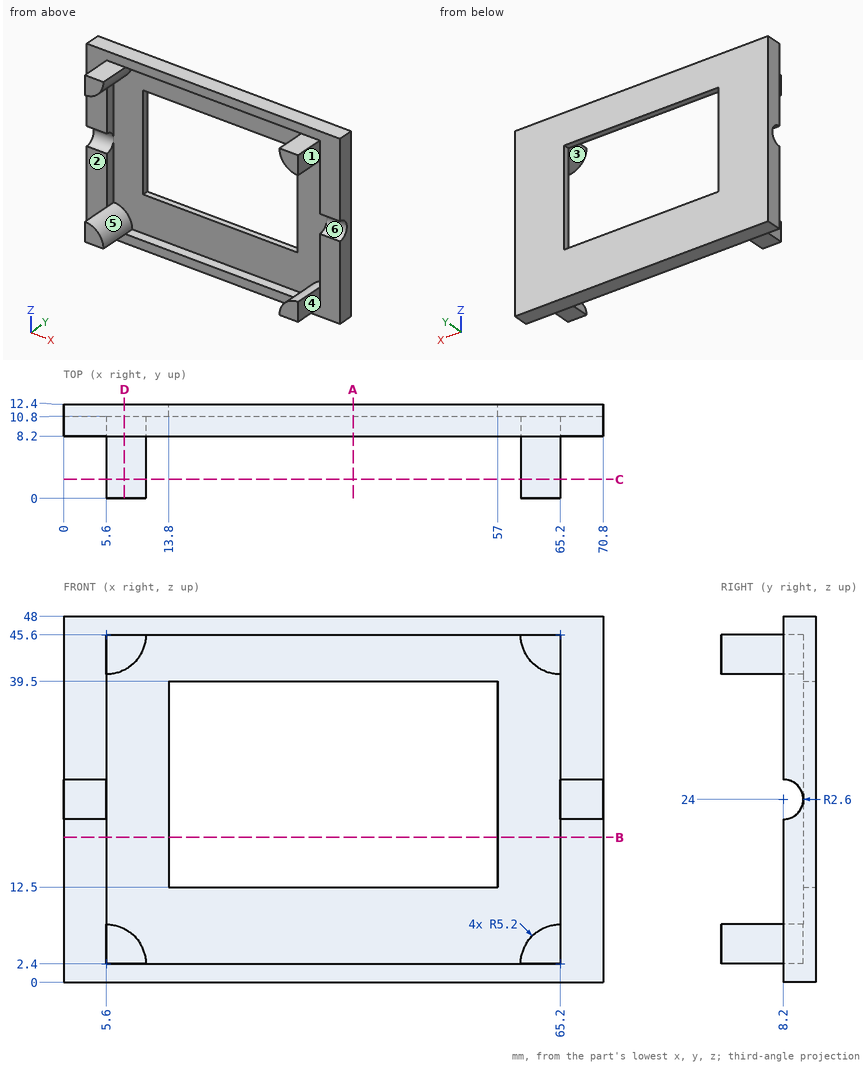
Geometry check sheet. Reference: drawing and pictorial views, mm from the part's lowest x, y, z. A direction names the side the tool comes from. Coordinates: 2 decimals unless noted, no trailing zeros. Loops run counter-clockwise (first coordinate to the right, second up) from the corner with the lowest first, then second, coordinate; pieces in that order, holes last.
1) Material ranges on probe 1 along X at (y, z) = (9.25, 29.5); probe 2 along Z at (x, y) = (44, 9.75); probe 3 along Y at (x, z) = (28, 8), recorded low to high.
2) Sectioned sample at C-C (y = 2.5). Record the boundary of the cut face in (x, z), and give its area (3 significant figures).
3) Sectioned sample at A-A (x = 38). Record the boundary of the cut face in (y, z).
4) Sectioned sample at D-D (x = 8). Record the boundary of the cut face in (y, z), and give its area (3 significant figures).
5) Access from +Z, -Z, +X, -X, +Y, -Y to the whole of each face (thin tool, end or side, straight path). Record for the marked faces 4, 5 and 6.
6) Gauge pin test, flat ends, axial feed: pin 1 (2.5 mm diameter, centred on x = 9, y = 3, fed in from +Z); pin 2 (6 mm diameter, centred on y = 5, z = 20.5, fed in from -X); pin 3 (2.5 mm diameter, centred on y = 4.5, z = 43.5, fed in from -X); pin 4 (17 mm diameter, centred on x = 23.5, z = 41.5, fed in from -Y). Record the tip position at first contact, or that the pin passes through.
7) Release check for a two-part mould opening along X. For the marked faces 1, 2 and 3 record: released by +X, released by -X, zero draft, split by the parting line, or undercut.
8) Sectioned sample at B-B (z = 19). Record the boundary of the cut face in (x, y).
Check sheet entries:
1. probe 1: x = 0 to 5.6, 65.2 to 70.8
1. probe 2: z = 0 to 2.4, 45.6 to 48
1. probe 3: y = 10.8 to 12.4
2. outline: (5.6, 2.4) - (10.8, 2.4) arc R5.2 ccw to (5.6, 7.6) - close; (5.6, 40.4) arc R5.2 ccw to (10.8, 45.6) - (5.6, 45.6) - close; (60, 2.4) - (65.2, 2.4) - (65.2, 7.6) arc R5.2 ccw to start; (60, 45.6) arc R5.2 ccw to (65.2, 40.4) - (65.2, 45.6) - close
2. area: 84.9 mm2
3. outline: (8.2, 0) - (12.4, 0) - (12.4, 12.5) - (10.8, 12.5) - (10.8, 2.4) - (8.2, 2.4) - close; (8.2, 45.6) - (10.8, 45.6) - (10.8, 39.5) - (12.4, 39.5) - (12.4, 48) - (8.2, 48) - close
4. outline: (0, 2.4) - (8.2, 2.4) - (8.2, 0) - (12.4, 0) - (12.4, 48) - (8.2, 48) - (8.2, 45.6) - (0, 45.6) - (0, 40.99) - (10.8, 40.99) - (10.8, 7.01) - (0, 7.01) - close
4. area: 189 mm2
5. face 4: +Z, -Z, +X, -Y
5. face 5: -Y
5. face 6: +X, -X, -Y
6. pin 1: stops at z = 45.6
6. pin 2: passes through
6. pin 3: stops at x = 5.6
6. pin 4: stops at y = 8.2
7. face 1: released by +X
7. face 2: zero draft
7. face 3: undercut
8. outline: (0, 8.2) - (5.6, 8.2) - (5.6, 10.8) - (13.8, 10.8) - (13.8, 12.4) - (0, 12.4) - close; (57, 10.8) - (65.2, 10.8) - (65.2, 8.2) - (70.8, 8.2) - (70.8, 12.4) - (57, 12.4) - close
